Work out the finished part from the listing and answer in its coordinate system (mm). Face numbers are marked on the shaded views. Coordinates: 2 decimals unless noted, no trailing zeros. Loops run counter-clockwise (first coordinate to the right, second up) from the corner with the lowest first, then second, coordinate; pieces in that order, holes last. Notation, with made-up numbers: (-31.5, 4) -> (9.5, 4) arc R29 cw to (9.5, 35) -> close; hole circle Ø7 at (48, 38). An arc over 180 degrees is marked (long way). One line per question, with ' | ' between items.
```python
from build123d import *

# Parameters (mm, degrees)
SKETCH1_R           = 1.5
BOSS_EXTRUDE1_DEPTH = 3
BOSS_EXTRUDE2_START = 51.5
BOSS_EXTRUDE2_DEPTH = 51.5
BOSS_EXTRUDE3_START = 54.5
SKETCH1_4_R         = 1.5
BOSS_EXTRUDE3_DEPTH = 3
FILLET1_R           = 2


with BuildPart() as part:
    # Sketch1 → Boss-Extrude1 (new body)
    # profile 1 of 4: a face of its own
    with BuildSketch(Plane(origin=(0, 0, 0), x_dir=(1, 0, 0), z_dir=(0, 1, 0))):
        with BuildLine():
            ThreePointArc((5, 50.854793284), (0, 51.1), (-5, 50.854793284))
            Line((-5, 50.854793284), (-5, 46.833855276))
            ThreePointArc((-5, 46.833855276), (0, 47.1), (5, 46.833855276))
            Line((5, 46.833855276), (5, 50.854793284))
        make_face()
    # profile 2 of 4: a face of its own
    with BuildSketch(Plane(origin=(0, 0, 0), x_dir=(1, 0, 0), z_dir=(0, 1, 0))):
        with BuildLine():
            ThreePointArc((5, 46.833855276), (0, 47.1), (-5, 46.833855276))
            Line((-5, 46.833855276), (-5, 38.778989157))
            ThreePointArc((-5, 38.778989157), (0, 39.1), (5, 38.778989157))
            Line((5, 38.778989157), (5, 46.833855276))
        make_face()
        with Locations((0, 42.5)):
            Circle(SKETCH1_R, mode=Mode.SUBTRACT)
    # profile 3 of 4: a face of its own
    with BuildSketch(Plane(origin=(0, 0, 0), x_dir=(1, 0, 0), z_dir=(0, 1, 0))):
        with Locations((0, 42.5)):
            Circle(SKETCH1_R)
    # profile 4 of 4: a face of its own
    with BuildSketch(Plane(origin=(0, 0, 0), x_dir=(1, 0, 0), z_dir=(0, 1, 0))):
        with BuildLine():
            ThreePointArc((5, 38.778989157), (0, 39.1), (-5, 38.778989157))
            Line((-5, 38.778989157), (-5, 15.198684154))
            ThreePointArc((-5, 15.198684154), (0, 16), (5, 15.198684154))
            Line((5, 15.198684154), (5, 38.778989157))
        make_face()
        with Locations(Location((0, 20, 0), (0, 0, 270))):
            Circle(SKETCH1_R, mode=Mode.SUBTRACT)
    extrude(amount=-BOSS_EXTRUDE1_DEPTH)

    # Sketch1_3 → Boss-Extrude2 (add)
    with BuildSketch(Plane(origin=(0, 0, 0), x_dir=(1, 0, 0), z_dir=(0, 1, 0)).offset(BOSS_EXTRUDE2_START)):
        with BuildLine():
            ThreePointArc((5, 50.854793284), (0, 51.1), (-5, 50.854793284))
            Line((-5, 50.854793284), (-5, 46.833855276))
            ThreePointArc((-5, 46.833855276), (0, 47.1), (5, 46.833855276))
            Line((5, 46.833855276), (5, 50.854793284))
        make_face()
    extrude(amount=-BOSS_EXTRUDE2_DEPTH)

    # Sketch1_4 → Boss-Extrude3 (add)
    # profile 1 of 2: a face of its own
    with BuildSketch(Plane(origin=(0, 0, 0), x_dir=(1, 0, 0), z_dir=(0, 1, 0)).offset(BOSS_EXTRUDE3_START)):
        with BuildLine():
            ThreePointArc((5, 46.833855276), (0, 47.1), (-5, 46.833855276))
            Line((-5, 46.833855276), (-5, 38.778989157))
            ThreePointArc((-5, 38.778989157), (0, 39.1), (5, 38.778989157))
            Line((5, 38.778989157), (5, 46.833855276))
        make_face()
        with Locations(Location((0, 42.5, 0), (0, 0, 270))):
            Circle(SKETCH1_4_R, mode=Mode.SUBTRACT)
    # profile 2 of 2: a face of its own
    with BuildSketch(Plane(origin=(0, 0, 0), x_dir=(1, 0, 0), z_dir=(0, 1, 0)).offset(BOSS_EXTRUDE3_START)):
        with BuildLine():
            ThreePointArc((5, 50.854793284), (0, 51.1), (-5, 50.854793284))
            Line((-5, 50.854793284), (-5, 46.833855276))
            ThreePointArc((-5, 46.833855276), (0, 47.1), (5, 46.833855276))
            Line((5, 46.833855276), (5, 50.854793284))
        make_face()
    extrude(amount=-BOSS_EXTRUDE3_DEPTH)

    # Fillet1
    fillet1_edges = [part.edges().sort_by_distance(p)[0] for p in [
        (5, -1.5, -15.198684154),
        (-5, -1.5, -15.198684154),
        (5, 53, -38.778989157),
        (-5, 53, -38.778989157),
    ]]
    fillet(fillet1_edges, radius=FILLET1_R)


solid = part.part
```
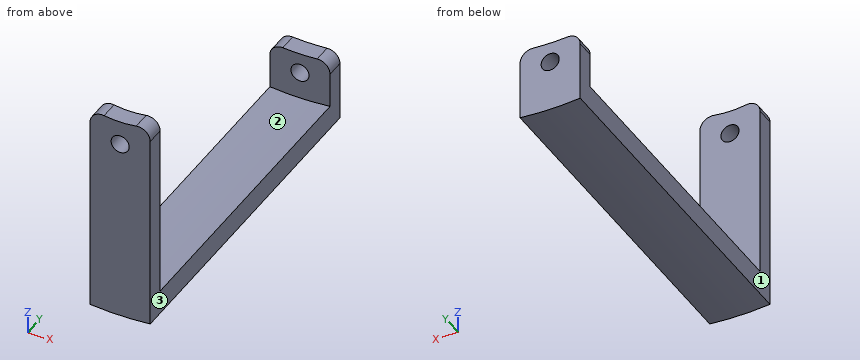
1) Find section B-B (x = 0). Write down the section's boundary in (y, z), plus the area to 3 significant figures.
Check values:
outline: (-3, -51.1) -> (54.5, -51.1) -> (54.5, -44) -> (51.5, -44) -> (51.5, -47.1) -> (0, -47.1) -> (0, -21.5) -> (-3, -21.5) -> close; (-3, -18.5) -> (0, -18.5) -> (0, -16) -> (-3, -16) -> close; (51.5, -41) -> (54.5, -41) -> (54.5, -39.1) -> (51.5, -39.1) -> close | area: 329 mm^2
2) Find section C-C (z = -20). Write down the section's boundary in (x, y).
Check values:
outline: (-5, -3) -> (-1.5, -3) -> (-1.5, 0) -> (-5, 0) -> close; (1.5, -3) -> (5, -3) -> (5, 0) -> (1.5, 0) -> close
3) Find section A-A (z = -42.5). Write down the section's boundary in (x, y), plus the area to 3 significant figures.
Check values:
outline: (-5, -3) -> (5, -3) -> (5, 0) -> (-5, 0) -> close; (-5, 51.5) -> (-1.5, 51.5) -> (-1.5, 54.5) -> (-5, 54.5) -> close; (1.5, 51.5) -> (5, 51.5) -> (5, 54.5) -> (1.5, 54.5) -> close | area: 51.0 mm^2
4) A flat-ended cylindrical pin translates along its axis: pin 1 (4 mm diameter, centred on x = 0, z = -20, fed in from +Y). Find the tip coordinate at first contact, or state that the pin passes through.
Check values:
pin 1: stops at y = 0
5) The mould has two halves that part along X. Classify the marked faces 1, 2 and 3: released by +X, released by -X, zero draft, split by the parting line, or undercut.
Check values:
face 1: released by -X | face 2: undercut | face 3: released by +X
6) Find the intervals of material crossed by line 1 along X through (y, z) = (-1, -20); line 2 along Y through (x, z) = (3.75, -41); line 3 along Z through (x, y) = (1, 50), in increasing order.
Check values:
line 1: x = -5 to -1.5, 1.5 to 5 | line 2: y = -3 to 0, 51.5 to 54.5 | line 3: z = -51.09 to -47.09
7) Find section D-D (x = -3.5). Write down the section's boundary in (y, z).
Check values:
outline: (-3, -50.98) -> (54.5, -50.98) -> (54.5, -39.05) -> (51.5, -39.05) -> (51.5, -46.97) -> (0, -46.97) -> (0, -15.81) -> (-3, -15.81) -> close
